```python
from build123d import *

# Parameters (mm, degrees)
F2_R     = 8.8916479932
F3_DEPTH = 7.62
F4_R     = 5.9660997996
F5_DEPTH = 33.782
F5_TAPER = 3
F6_R     = 23.449689891
F7_R     = 2.6928021488
F8_DEPTH = 6.1976
F9_R     = 6.2931418715


with BuildPart() as f1:
    # F0 (on Front) → F1 (revolve)
    with BuildSketch(Plane.XZ):
        Polygon((0, 8.7555544451), (0, -137.0834410191), (4.0525886504, -137.0834410191), (8.9142937213, -128.5754448824), (8.9142937213, -111.652046442), (7.8642298467, -111.652046442), (7.8642298467, -94.0267377846), (14.0556832775, -87.4014794827), (14.0556832775, -85.3735804558), (13.9548806474, -85.3735804558), (13.9548806474, -85.292108357), (14.0556832775, -85.292108357), (14.0556832775, -83.7196558714), (13.9222918078, -83.7196558714), (13.9222918078, -83.6381837726), (14.0556832775, -83.6381837726), (14.0556832775, -79.1663005948), (14.0252374113, -79.1663005948), (14.0252374113, -79.1377872229), (14.0556832775, -79.1377872229), (14.0556832775, -73.0870887637), (13.9991957694, -73.0870887637), (13.9991957694, -73.0259865522), (14.0556832775, -73.0259865522), (14.0556832775, -67.7627697587), (14.0434103087, -67.7627697587), (14.0434103087, -67.7536055446), (14.0556832775, -67.7536055446), (14.0556832775, -63.0693808198), (16.8571081012, -34.9119342864), (16.8571081012, -32.956559211), (16.7896877974, -32.956559211), (16.7896877974, -32.9383201897), (16.8571081012, -32.9383201897), (16.8571081012, -12.5459134579), (15.2300363407, 8.7555544451), align=None)
    revolve(axis=Axis((0, 0, -64.163943287), (0, 0, -1)))

    # F2 (on face) → F3 (join)
    with BuildSketch(Plane.XY.offset(8.7555544451)):
        Circle(F2_R)
    extrude(amount=F3_DEPTH)

    # F4 (on face) → F5 (join)
    with BuildSketch(Plane.XY.offset(16.3755544451)):
        Circle(F4_R)
    extrude(amount=F5_DEPTH, taper=F5_TAPER)

    # F6
    f6_edges = [f1.edges().sort_by_distance(p)[0] for p in [
        (-8.914294, 0, -128.575445),
    ]]
    fillet(f6_edges, radius=F6_R)

    # F7 (on face) → F8 (join)
    with BuildSketch(Plane(origin=(0, 0, -137.0834410191), x_dir=(1, 0, 0), z_dir=(0, 0, -1))):
        Circle(F7_R)
    extrude(amount=-F8_DEPTH)

    # F9
    f9_edges = [f1.edges().sort_by_distance(p)[0] for p in [
        (-15.230036, 0, 8.755554),
    ]]
    fillet(f9_edges, radius=F9_R)


solid = f1.part
```
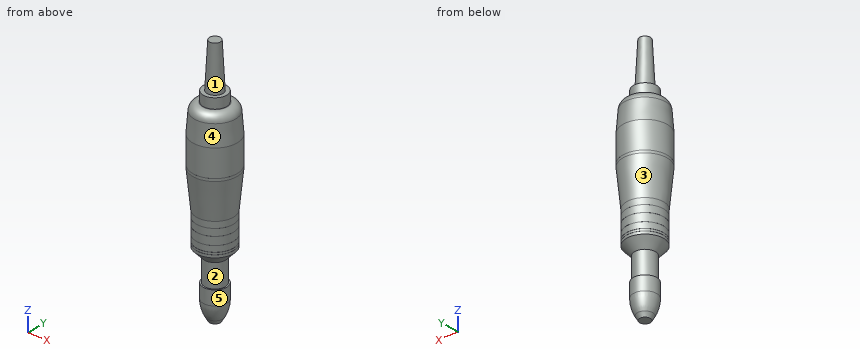
Can you work these out from the model? Positions are in its coordinate system, mm. Face numbers are marked on the shaded views. A direction names the side the tool comes from. Round coordinates to 2 decimals unless told otherwise and drop trailing zeros. Loops run counter-clockwise (first coordinate to the right, second up) from the corner with the lowest first, then second, coordinate; pieces in that order, holes last. Notation, with made-up numbers: (11, -13.5) -> (63, -13.5) arc R21 ccw to (63, 13.5) -> close; hole circle Ø3 at (-14, 48.5). An arc over 180 degrees is marked (long way). One line per item, written item: value. Start each with the question number.
1. If I drill on probe 1 along X at (y, z) = (4.5, 6); probe 2 along X at (y, z) = (-14, -28.5); probe 3 along Z at (x, y) = (-2, 9), over which ranges is the centre line in solid material (lowest first)?
2. For pin 1 (10 mm diameter, centred on x = 10, y = -12.5, fed in from -Z); pin 2 (1 mm diameter, centred on y = 7.5, z = -37.5, fed in from -X); pin 3 (3 mm diameter, centred on x = 11.5, y = 8.5, fed in from -Z), each with a flat end and sliding along its axis, tell me the tip position at first contact or that it passes through.
3. For the marked faces 4 and 5, which set-ups out of +Z, -Z, +X, -X, +Y, -Y let a thin tool reach every point of the face, with its end or its side?
4. If we section it at A-A, the plane z = -52.5: Write out the boundary of the cut face in (x, y), then the cut area to 3 significant figures.
5. If we mould it in two halves opening along Z, with no side actions, what happens to the marked faces 1, 2 and 3? For each: pulls with the +Z half, pulls with the -Z half, needs draft (parallel to the pull), parting line crosses it, or undercut.
Calculated:
1. probe 1: x = -13.89 to 13.89
1. probe 2: x = -9.39 to 9.39
1. probe 3: z = -92.58 to 8.76
2. pin 1: stops at z = -90.66
2. pin 2: stops at x = -15.06
2. pin 3: stops at z = -88.74
3. face 4: +Z
3. face 5: -Z
4. outline: circle Ø30.21 at (0, 0)
4. area: 717 mm²
5. face 1: pulls with the +Z half
5. face 2: undercut
5. face 3: pulls with the -Z half
